```python
from build123d import *

# Parameters (mm, degrees)
BOSS_EXTRUDE1_DEPTH     = 19.05
BOSS_EXTRUDE1_DRAFT     = -29.54735891
CUT_EXTRUDE1_DEPTH      = 374.741958864
CUT_EXTRUDE1_DEPTH_BACK = 374.741958864
SKETCH2_OUTSIDE_W       = 447.362
SKETCH2_OUTSIDE_H       = 98.57
SKETCH2_OUTSIDE_W_2     = 346.244171738
SKETCH2_OUTSIDE_H_2     = 100.341978652
CUT_EXTRUDE2_DEPTH      = 364.132941986


with BuildPart() as part:
    # Sketch1 → Boss-Extrude1 (with draft: the straight prism first)
    with BuildSketch(Plane(origin=(0, 0, 0), x_dir=(1, 0, 0), z_dir=(0, 1, 0))):
        Polygon((0, 0), (0, -96.93730792), (346.244171738, -63.94360396), (346.244171738, -32.99370396), align=None)
    extrude(amount=BOSS_EXTRUDE1_DEPTH)
    # Boss-Extrude1: the draft: its side faces are tilted about the plane it starts from
    boss_extrude1_sides = [part.faces().sort_by_distance(p)[0] for p in [
        (0, 9.525, 48.46865396),
        (173.122085869, 9.525, 80.44045594),
        (346.244171738, 9.525, 48.46865396),
        (173.122085869, 9.525, 16.49685198),
    ]]
    draft(boss_extrude1_sides, Plane(origin=(0, 0, 0), x_dir=(1, 0, 0), z_dir=(0, 1, 0)), BOSS_EXTRUDE1_DRAFT)

    # Sketch2 outside → Cut-Extrude1 (cut, two sides: drawn at the far end of the back side and taken through both)
    with BuildSketch(Plane.XY.offset(-CUT_EXTRUDE1_DEPTH_BACK)):
        with Locations((173.122, 9.525)):
            Rectangle(SKETCH2_OUTSIDE_W, SKETCH2_OUTSIDE_H)
        with Locations((173.122085869, 50.170989326)):
            Rectangle(SKETCH2_OUTSIDE_W_2, SKETCH2_OUTSIDE_H_2, mode=Mode.SUBTRACT)
    extrude(amount=CUT_EXTRUDE1_DEPTH + CUT_EXTRUDE1_DEPTH_BACK, mode=Mode.SUBTRACT)

    # Sketch3 → Cut-Extrude2 (cut, through all)
    with BuildSketch(Plane.XY):
        Polygon((320.844171738, 0), (320.844171738, 9.525), (346.244171738, 13.775502271), (346.244171738, 0), align=None)
    extrude(amount=CUT_EXTRUDE2_DEPTH, mode=Mode.SUBTRACT)


solid = part.part
```
Here's how the part is built. I have some questions about the finished solid (model axes, mm). A direction names the side the tool comes from. Round coordinates to 2 decimals unless told otherwise and drop trailing zeros. Loops run counter-clockwise (first coordinate to the right, second up) from the corner with the lowest first, then second, coordinate; pieces in that order, holes last. Notation, with made-up numbers: (39, 32.25) -> (90, 32.25) arc R17 cw to (90, 52.25) -> close; hole circle Ø11 at (-20, 55.25). An arc over 180 degrees is marked (long way). Answer as CSV lines item,"result". Start each with the question number.
1. Imagine slicing it at C-C on y = 4.25. Write out the boundary of the cut face in (x, z).
2. Imagine slicing it at D-D on z = -3. Write out the boundary of the cut face in (x, y).
3. I need wall thicknesses on probe 1 along X at (y, z) = (4.25, 31); probe 2 along Z at (x, y) = (309, 2.5); probe 3 along Z at (x, y) = (87.5, 7). Which ranges of each line are inside material? Lowest first, please. Write a range as from..to.
4. Imagine slicing it at B-B on x = 233.5. Write out the boundary of the cut face in (y, z), plus the area to 3 significant figures.
5. I'm going to push flat-ended pins straight in: P1, Ø2, axis at x = 89, y = 16.5, coming from the -Z side; P2, Ø2, axis at x = 281.5, y = 12.5, coming from the -Z side; P3, Ø5, axis at x = 242.5, y = 14, coming from the +Z side. Where does each tip first touch, or does it pass through?
6. For faces 1 (the face through (132, 19.05, 48)), 2 (the face through (320.844, 5, 48)), which set-ups out of +Z, -Z, +X, -X, +Y, -Y let a thin tool reach every point of the face, with its end or its side?
Solution:
1,outline,"(0, -2.42) -> (320.84, 28.15) -> (320.84, 68.78) -> (0, 99.36) -> close"
2,outline,"(0, 5.27) -> (82.36, 19.05) -> (0, 19.05) -> close"
3,probe 1,"0..320.84"
3,probe 2,"28.02..68.92"
3,probe 3,"4.35..92.59"
4,outline,"(0, 22.25) -> (19.05, 11.4) -> (19.05, 85.53) -> (0, 74.69) -> close"
4,area,"1,210 mm²"
5,P1,"z = -1.49"
5,P2,"z = 19.13"
5,P3,"z = 83.24"
6,face 1,"+Z, -Z, +X, -X, +Y"
6,face 2,"+Z, -Z, +X, -Y"
